```python
from build123d import *

# Parameters (mm, degrees)
SKETCH_2_R               = 9
CUT_EXTRUDE_2_DEPTH      = 132.742172443
PATTERN_CIRCULAR_2_COUNT = 4
EXTRUDE_START            = 2
SKETCH_3_R               = 61.5
SKETCH_3_R_2             = 37.5
EXTRUDE_1_DEPTH          = 2
CHAMFER_5_SIZE           = 1.5


with BuildPart() as part:
    # Sketch 1 → Revolve 1 (revolve)
    with BuildSketch(Plane.XY, mode=Mode.PRIVATE) as revolve_1_sk:
        Polygon((-34, 37.5), (0, 37.5), (0, 90), (-15, 90), (-15, 44.7), (-34, 44.7), align=None)
    revolve(revolve_1_sk.sketch.rotate(Axis((0, 0, 0), (-1, 0, 0)), 90), axis=Axis((0, 0, 0), (-1, 0, 0)))

    # Sketch 2 → Cut-Extrude 2 (cut, through all)
    with BuildSketch(Plane(origin=(0, 0, 0), x_dir=(0, 0, -1), z_dir=(1, 0, 0))):
        with Locations((0, 72.5)):
            Circle(SKETCH_2_R)
    cut_extrude_2 = extrude(amount=-CUT_EXTRUDE_2_DEPTH, mode=Mode.SUBTRACT)

    # Pattern Circular 2: Cut-Extrude 2 ×4 about axis
    pattern_circular_2_axis = Axis((0, 0, 0), (1, 0, 0))
    for i in range(1, PATTERN_CIRCULAR_2_COUNT):
        add(cut_extrude_2.rotate(pattern_circular_2_axis, i * 360 / PATTERN_CIRCULAR_2_COUNT), mode=Mode.SUBTRACT)

    # Sketch 3 → Extrude 1 (add)
    with BuildSketch(Plane(origin=(0, 0, 0), x_dir=(0, 0, -1), z_dir=(1, 0, 0)).offset(EXTRUDE_START)):
        Circle(SKETCH_3_R)
        Circle(SKETCH_3_R_2, mode=Mode.SUBTRACT)
    extrude(amount=-EXTRUDE_1_DEPTH)

    # Chamfer 5
    chamfer_5_edges = [part.edges().sort_by_distance(p)[0] for p in [
        (2, 0, 61.5),
    ]]
    chamfer(chamfer_5_edges, length=CHAMFER_5_SIZE)


solid = part.part
```
Input: part model. Units: mm. Frame: model coordinates. A direction names the side the tool comes from. Round coordinates to 2 decimals unless told otherwise and drop trailing zeros. Write each loop counter-clockwise with the first axis right and the second up, starting at its lowest first coordinate (ties: lowest second). Pieces come first, ordered by that corner, then holes. Notation, with made-up numbers: (44, -20) -> (70, -20) arc R24 ccw to (70, -1) -> close; hole circle Ø10 at (36.5, 6). An arc over 180 degrees is marked (long way). Answer as CSV lines item,"result".
1. Reachability of faces 5 (the cylindrical face through (-24.63, -44.32, 5.82)), 6 (the cylindrical face through (0.25, -54.56, -28.38)), 7 (the flat face through (2, -26, 28)) from +Z, -Z, +X, -X, +Y, -Y: full face, straight path, thin tool, end or side. Return the list, or none.
Geometry says:
face 5,"-X"
face 6,"+X"
face 7,"+Z, -Z, +X, +Y, -Y"
2. Mould query, pull axis Z, two halves, no side actions, for faces 1 (the cylindrical face through (-7.605, 79.845, -41.53)), 2 (the cylindrical face through (-7.395, -1.951, 63.714)), 3 (the cylindrical face through (-7.395, 63.714, 1.951)), 4 (the flat face through (-15, 19, 41)). Classes: +Z half, -Z half, draft (parallel to the pull), parting line (faces both ways), or undercut.
Geometry says:
face 1,"parting line"
face 2,"undercut"
face 3,"undercut"
face 4,"draft"
3. Ray query, L1, parallel to Y at x = -11.5, z = -0.5; L2, parallel to Y at x = -6.5, z = 4; L3, parallel to Y at x = -3.5, z = -15. Return the intervals inside material, ascending. Write a range as [from, to].
Geometry says:
L1,"y = [-90, -81.49], [-63.51, -37.5], [37.5, 63.51], [81.49, 90]"
L2,"y = [-89.91, -80.56], [-64.44, -37.29], [37.29, 64.44], [80.56, 89.91]"
L3,"y = [-88.74, -34.37], [34.37, 88.74]"
4. Section A-A (z = 0). Return the cut outline in (x, y), plus the area to 3 significant figures.
Geometry says:
outline,"(-34, -44.7) -> (-15, -44.7) -> (-15, -63.5) -> (0, -63.5) -> (0, -61.5) -> (0.5, -61.5) -> (2, -60) -> (2, -37.5) -> (-34, -37.5) -> close; (-34, 37.5) -> (2, 37.5) -> (2, 60) -> (0.5, 61.5) -> (0, 61.5) -> (0, 63.5) -> (-15, 63.5) -> (-15, 44.7) -> (-34, 44.7) -> close; (-15, -90) -> (0, -90) -> (0, -81.5) -> (-15, -81.5) -> close; (-15, 81.5) -> (0, 81.5) -> (0, 90) -> (-15, 90) -> close"
area,"1,400 mm^2"
5. Section C-C (x = -11). Return the cut outline in (y, z), plus the area to 3 significant figures.
Geometry says:
outline,"circle Ø180 at (0, 0); hole circle Ø18 at (-72.5, 0); hole circle Ø75 at (0, 0); hole circle Ø18 at (0, -72.5); hole circle Ø18 at (0, 72.5); hole circle Ø18 at (72.5, 0)"
area,"20,000 mm^2"
6. Contact query for flat-ended pins moving along their axis: P1, Ø4, axis at y = -56.5, z = -41, coming from the +X side; P2, Ø3, axis at x = -9.5, z = 6, coming from the +Y side; P3, Ø2, axis at x = -6, y = 31.5, coming from the +Z side; P4, Ø11, axis at y = 72.5, z = 0, coming from the +X side. Output: stop coordinate, or through.
Geometry says:
P1,"stops at x = 0"
P2,"stops at y = 89.89"
P3,"stops at z = 84.67"
P4,"passes through"
7. Section B-B (z = 72.5). Return the cut outline in (x, y).
Geometry says:
outline,"(-15, -53.33) -> (0, -53.33) -> (0, -9) -> (-15, -9) -> close; (-15, 9) -> (0, 9) -> (0, 53.33) -> (-15, 53.33) -> close"
